The listing builds one solid part. Answer for the finished solid, in the listing's coordinates (mm). A direction names the side the tool comes from. Round coordinates to 2 decimals unless told otherwise and drop trailing zeros. Loops run counter-clockwise (first coordinate to the right, second up) from the corner with the lowest first, then second, coordinate; pieces in that order, holes last. Notation, with made-up numbers: (86.5, -23) -> (95.5, -23) arc R24 cw to (95.5, 6) -> close; hole circle Ø2 at (2, 42.25). An arc over 180 degrees is marked (long way). Answer in a Markdown table with one row per item. Add a question column.
```python
from build123d import *

# Parameters (mm, degrees)
SKETCH002_R  = 1.8
PAD002_DEPTH = 3
SKETCH003_R  = 10
PAD003_DEPTH = 65
PAD004_DEPTH = 20
SKETCH008_R  = 6
POCKET_DEPTH = 39


with BuildPart() as part:
    # Sketch002 → Pad002 (new body)
    with BuildSketch(Plane.XY):
        with BuildLine():
            Line((120, 0), (10, 0))
            ThreePointArc((0, 10), (2.928932, 2.928932), (10, 0))
            Line((0, 35), (0, 10))
            ThreePointArc((5, 40), (1.464466, 38.535534), (0, 35))
            Line((125, 40), (5, 40))
            ThreePointArc((130, 35), (128.535534, 38.535534), (125, 40))
            Line((130, 10), (130, 35))
            ThreePointArc((120, 0), (127.071068, 2.928932), (130, 10))
        make_face()
        with Locations((120, 34)):
            Circle(SKETCH002_R, mode=Mode.SUBTRACT)
        with Locations((10, 34)):
            Circle(SKETCH002_R, mode=Mode.SUBTRACT)
        with Locations((65, 34)):
            Circle(SKETCH002_R, mode=Mode.SUBTRACT)
    extrude(amount=-PAD002_DEPTH)

    # Sketch003 → Pad003 (join)
    with BuildSketch(Plane.XY.offset(-3)):
        with Locations((10, 10)):
            Circle(SKETCH003_R)
        with Locations((120, 10)):
            Circle(SKETCH003_R)
    extrude(amount=-PAD003_DEPTH)

    # Sketch004 → Pad004 (join)
    with BuildSketch(Plane.XZ):
        with BuildLine():
            Line((10, -3), (120, -3))
            Line((120, -3), (120, -23))
            ThreePointArc((120, -23), (115.606602, -12.393398), (105, -8))
            Line((25, -8), (105, -8))
            ThreePointArc((25, -8), (14.393398, -12.393398), (10, -23))
            Line((10, -23), (10, -3))
        make_face()
    extrude(amount=-PAD004_DEPTH)

    # Sketch008 → Pocket (cut)
    with BuildSketch(Plane.XY.offset(-68)):
        with Locations((10, 10)):
            Circle(SKETCH008_R)
        with Locations((120, 10)):
            Circle(SKETCH008_R)
    extrude(amount=POCKET_DEPTH, mode=Mode.SUBTRACT)

    # Cone001 → Cone001 (revolve, cut)
    with BuildSketch(Plane(origin=(10, 10, -29), x_dir=(1, 0, 0), z_dir=(0, -1, 0))):
        Polygon((0, 0), (6, 0), (0, 10), align=None)
    revolve(axis=Axis((10, 10, -29), (0, 0, 1)), mode=Mode.SUBTRACT)

    # Cone002 → Cone002 (revolve, cut)
    with BuildSketch(Plane(origin=(120, 10, -29), x_dir=(1, 0, 0), z_dir=(0, -1, 0))):
        Polygon((0, 0), (6, 0), (0, 10), align=None)
    revolve(axis=Axis((120, 10, -29), (0, 0, 1)), mode=Mode.SUBTRACT)


solid = part.part
```
Item 1: Section C-C, the plane z = -31 is taken. Write down the section's boundary in (x, y).
Item 2: Section D-D, the plane x = 40 is taken. Write down the section's boundary in (y, z).
Item 3: For faces 4 (the cylindrical face through (129, 38, -1)), 5 (the flat face through (64, 10, -8)), 6 (the cylindrical face through (21.171, 10.694, -8.497)), determine the directions among +Z, -Z, +X, -X, +Y, -Y from which every point of the face is accessible in a straight line to the end or side of a thin tool.
Item 4: The mould has two halves that part along X. Classify faces 1 (the cylindrical face through (9.766, 35.785, -1.479)), 2 (the flat face through (65, 20, -7)), 3 (the flat face through (0, 23, -1)): +X half, -X half, draft (parallel to the pull), parting line (faces both ways), or undercut.
Item 5: Section B-B, the plane z = -12 is taken. Write down the section's boundary in (x, y).
Item 6: Section A-A, the plane x = 65 is taken. Write down the section's boundary in (y, z).
Item 7: Consider L1, parallel to Y at x = 120, z = -2.1; L2, parallel to Y at x = 120, z = -45.5; L3, parallel to X at y = 7, z = -58.5. Determine where each line is inside the solid, lowest interval first. Write a range as from..to.
Item 8: Flat-ended cylindrical pins translate along their axes: P1, Ø2, axis at x = 65, y = 34, coming from the -Z side; P2, Ø1.5, axis at y = 5.5, z = -25, coming from the -X side; P3, Ø8, axis at y = 5, z = -44, coming from the -X side; P4, Ø4, axis at x = 15, z = -45, coming from the +Y side. Find the tip coordinate at first contact, or state that the pin passes through.
Here are the results:
| question | item | result |
|---|---|---|
| 1 | outline | circle Ø20 at (10, 10); circle Ø20 at (120, 10); hole circle Ø12 at (10, 10); hole circle Ø12 at (120, 10) |
| 2 | outline | (0, -8) -> (20, -8) -> (20, -3) -> (40, -3) -> (40, 0) -> (0, 0) -> close |
| 3 | face 4 | +Z, -Z, +X, +Y |
| 3 | face 5 | -Z, +Y, -Y |
| 3 | face 6 | -Z |
| 4 | face 1 | undercut |
| 4 | face 2 | draft |
| 4 | face 3 | -X half |
| 5 | outline | (10, 0) -> (14.8, 0) -> (14.8, 1.23) arc R10 ccw to (14.8, 18.77) -> (14.8, 20) -> (10, 20) arc R10 ccw to start; (115.2, 0) -> (120, 0) arc R10 ccw to (120, 20) -> (115.2, 20) -> (115.2, 18.77) arc R10 ccw to (115.2, 1.23) -> close |
| 6 | outline | (0, -8) -> (20, -8) -> (20, -3) -> (32.2, -3) -> (32.2, 0) -> (0, 0) -> close; (35.8, -3) -> (40, -3) -> (40, 0) -> (35.8, 0) -> close |
| 7 | L1 | y = 0..32.2, 35.8..40 |
| 7 | L2 | y = 0..4, 16..20 |
| 7 | L3 | x = 0.46..4.8, 15.2..19.54, 110.46..114.8, 125.2..129.54 |
| 8 | P1 | passes through |
| 8 | P2 | stops at x = 0.73 |
| 8 | P3 | stops at x = 0.05 |
| 8 | P4 | stops at y = 19.54 |
